Verification items for this drawing (mm, ordinates from the low corner). Round coordinates to 2 decimals unless told otherwise and drop trailing zeros. Use a Markdown table: item, result. Add a question column.
Item 1: Material ranges on probe 1 along Z at (x, y) = (21.5, 266.7), recorded low to high. Write a range as [from, to].
Item 2: Gauge pin test, flat ends, axial feed: pin 1 Ø3 at (x, y) = (12.7, 241.3) entering from -Z; pin 2 Ø3 at (x, z) = (7, 19) entering from -Y. Record the tip position at first contact, or that the pin passes through.
Item 3: Sectioned sample at A-A, the plane x = 3. State how many separate pieces and enclosed holes the cut face has, and give its area (3 significant figures).
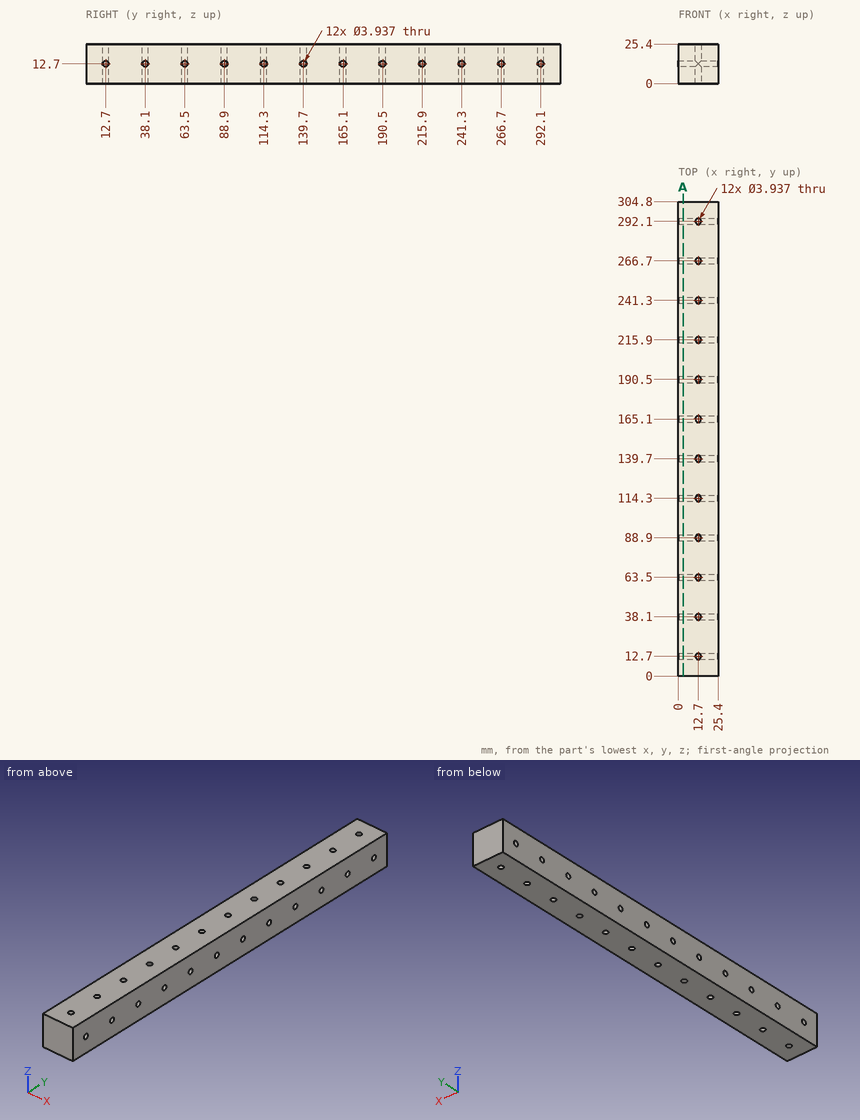
Found:
| question | item | result |
|---|---|---|
| 1 | probe 1 | z = [0, 10.73], [14.67, 25.4] |
| 2 | pin 1 | passes through |
| 2 | pin 2 | stops at y = 0 |
| 3 | separate pieces | 1 |
| 3 | enclosed holes | 12 |
| 3 | area | 7,600 mm2 |
